Work out the finished part from the listing and answer in its coordinate system (mm). A direction names the side the tool comes from. Round coordinates to 2 decimals unless told otherwise and drop trailing zeros. Loops run counter-clockwise (first coordinate to the right, second up) from the corner with the lowest first, then second, coordinate; pieces in that order, holes last. Notation, with made-up numbers: M 55,54.5 L 61,54.5 A27 cw 61,78.5 Z; hole C 88.5,13.25 d4. An arc over 180 degrees is marked long. One line per item, written item: value.
Autodesk Fusion 360 part; units mm, degrees
sketch "Sketch2" plane through (0, 0, 0) normal (0, 0, 1) x (1, 0, 0)
  line L0 (33, -21) -> (-33, -21)
  line L1 (-33, -21) -> (-33, 21)
  line L2 (-33, 21) -> (33, 21)
  line L3 (33, 21) -> (33, -21)
  line L4 (33, -21) -> (-33, 21) construction
  line L5 (-33, -21) -> (33, 21) construction
  dimension "d1" = 66
  dimension "d2" = 42
extrude "Extrude1" add sketch "Sketch2" along normal blind 12
chamfer "Chamfer1" distance 12 angle 45 2 edges at (33, -21, 6) (33, 21, 6)
sketch "Sketch3" plane through (0, 0, 12) normal (0, 0, 1) x (-1, 0, 0)
  line L0 (-33, -9) -> (-21, -21)
  line L1 (-21, -21) -> (33, -21)
  line L2 (33, -21) -> (33, 21)
  line L3 (33, 21) -> (-21, 21)
  line L4 (-21, 21) -> (-33, 9)
  line L5 (-33, 9) -> (-33, -9)
  line L6 (33, -21) -> (21, -21)
  line L7 (21, -21) -> (21, 21)
  line L8 (21, 21) -> (33, 21)
  line L9 (33, 21) -> (33, -21)
  dimension "d6" = 12
extrude "Extrude2" add sketch "Sketch3" along normal blind 48 contours L1 L2 L3 L6 L7 L8 L9
fillet "Fillet1" radius 21 2 edges at (-27, -21, 60) (-27, 21, 60)
sketch "Sketch4" plane through (0, 0, 0) normal (0, 1, 0) x (1, 0, 0)
  line L0 (-21.1838, -54.3604) -> (-21.1838, -12.3604)
  line L1 (-21.1838, -12.3604) -> (32.8162, -12.3604)
  line L2 (-21.1838, -54.3604) -> (32.8162, -12.3604)
  dimension "d11" = 42
  dimension "d12" = 54
extrude "Extrude3" add sketch "Sketch4" along normal mid plane 12
equation "d12 = 66 mm - 12 mm"
1) Find the intervals of material crossed by probe 1 along X at (y, z) = (12, 29.5); probe 2 along Z at (x, y) = (23.5, 9.5); probe 3 along Y at (x, z) = (7, 16), in increasing order. Write a range as from..to.
Check values:
probe 1: -33..-21
probe 2: 0..12
probe 3: -6..6
2) For faces 1 (the face through (0, 6, 28)), 2 (the face through (6, 0, 12)), 3 (the face through (0, -6, 28)), determine the directions among +Z, -Z, +X, -X, +Y, -Y from which every point of the face is accessible in a straight line to the end or side of a thin tool.
Check values:
face 1: +Z, +X, +Y
face 2: +X, +Y, -Y
face 3: +Z, +X, -Y
3) Find section B-B (z = 40). Give the vertices of the cut face in (x, y).
Check values:
outline: M -33,-20.98 L -21,-20.98 L -21,-6 L -2.72,-6 L -2.72,6 L -21,6 L -21,20.98 L -33,20.98 Z
4) Find section C-C (y = -1). Give the vertices of the cut face in (x, z), then the cut area to 3 significant figures.
Check values:
outline: M -33,0 L 33,0 L 33,12 L -21,12 L -21,12.36 L 32.82,12.36 L -21,54.22 L -21,59.98 L -33,59.98 Z
area: 2,490 mm2
5) Find section A-A (x = -11). Give the vertices of the cut face in (y, z).
Check values:
outline: M -21,0 L 21,0 L 21,12 L -21,12 Z; M -6,12.36 L 6,12.36 L 6,46.44 L -6,46.44 Z
6) The mould has two halves that part along Z. Classify faces 4 (the face through (27, -15, 6)), 5 (the face through (0, 0, 0)), 6 (the face through (6, 0, 12.36)): +Z half, -Z half, draft (parallel to the pull), parting line (faces both ways), or undercut.
Check values:
face 4: draft
face 5: -Z half
face 6: undercut
7) Each of these flat-tipped pins is pushed along its axis until it touches: pin 1 (12.5 mm diameter, centred on x = 12, y = -9, fed in from +Z); pin 2 (10 mm diameter, centred on x = 4.5, z = 36, fed in from +Y); pin 3 (1.5 mm diameter, centred on x = 14.5, y = -9, fed in from +Z). Where does it stop, or does it pass through?
Check values:
pin 1: z = 32.82
pin 2: y = 6
pin 3: z = 12
